from build123d import *

# Parameters (mm, degrees)
F1_DEPTH = 96.012
F3_D     = 15.875
F3_DEPTH = 31.75
F3_TIP   = 4.7693311635
F5_DEPTH = 56.897
F6_W     = 28.956
F6_H     = 13.716
F6_W_2   = 25.4
F6_H_2   = 19.304
F7_DEPTH = 50.801
F9_DEPTH = 56.897


with BuildPart() as f1:
    # F0 (on Right) → F1 (new body)
    with BuildSketch(Plane.YZ):
        Polygon((55.828121284, -27.6095795721), (55.828121284, 23.1904204279), (43.128121284, 23.1904204279), (-1.067878716, -21.0055795721), (-1.067878716, -27.6095795721), align=None)
    extrude(amount=F1_DEPTH)

    # F3
    with Locations(Plane.YZ.offset(96.012)):
        with Locations((36.524121284, -11.8615795721)):
            Hole(F3_D / 2, depth=F3_DEPTH)
            with Locations((0, 0, -(F3_DEPTH + F3_TIP / 2))):  # 118° drill point
                Cone(0, F3_D / 2, F3_TIP, mode=Mode.SUBTRACT)

    # F4 (on face) → F5 (cut, through all)
    with BuildSketch(Plane(origin=(0, 55.828121284, 0), x_dir=(-1, 0, 0), z_dir=(0, 1, 0))):
        Polygon((-96.012, 4.3944204279), (-77.216, 23.1904204279), (-96.012, 23.1904204279), align=None)
    extrude(amount=-F5_DEPTH, mode=Mode.SUBTRACT)

    # F6 (on face) → F7 (cut, through all)
    with BuildSketch(Plane(origin=(0, 0, -27.6095795721), x_dir=(1, 0, 0), z_dir=(0, 0, -1))):
        with Locations((39.878, -5.790121284)):
            Rectangle(F6_W, F6_H)
        with Locations((83.312, -8.584121284)):
            Rectangle(F6_W_2, F6_H_2)
    extrude(amount=-F7_DEPTH, mode=Mode.SUBTRACT)

    # F8 (on face) → F9 (cut, through all)
    with BuildSketch(Plane(origin=(0, 55.828121284, 0), x_dir=(-1, 0, 0), z_dir=(0, 1, 0))):
        Polygon((-16.2123730209, 4.3944204279), (0, 4.3944204279), (0, 23.1904204279), (-48.768, 23.1904204279), align=None)
    extrude(amount=-F9_DEPTH, mode=Mode.SUBTRACT)


solid = f1.part
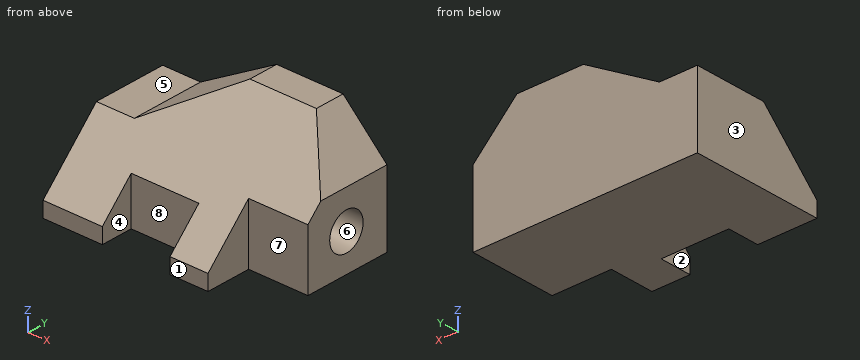
Build history of the part. All positions in model axes, mm. Face numbers are marked on the shaded views. A direction names the side the tool comes from. Give positions to 0.01 mm unless a question says otherwise; leave off trailing zeros. Order: outer loops, then holes, each group sorted by start corner. A loop starts at its lowest first (then second) coordinate and runs counter-clockwise, first axis right, second up. Notation, with made-up numbers: M 82.25,7.5 L 133.25,7.5 A21 cw 133.25,26.5 Z; hole C 43.5,15 d11. An arc over 180 degrees is marked long. Use one line per item in the form item = value.
Q1. Slice it at A-A, the plane y = 48. Write the cut outline in (x, z), and give its area (3 significant figures).
Conclusion:
outline = M 0,-27.61 L 96.01,-27.61 L 96.01,4.39 L 77.22,23.19 L 48.77,23.19 L 16.21,4.39 L 0,4.39 Z
area = 4,090 mm2
Q2. Pin check, flat tips, straight feed: P1, Ø10, axis at x = 61.5, z = 14.5, coming from the -Y side; P2, Ø18, axis at x = 11.5, y = 40, coming from the +Z side; P3, Ø6, axis at y = 35, z = 7.5, coming from the +X side. Stop position of each tip, or through.
Conclusion:
P1 = 29.44
P2 = 6.87
P3 = 95.91
Q3. Slice it at C-C, the plane x = 66. Write the cut outline in (y, z) (1 decimal).
Conclusion:
outline = M -1.1,-27.6 L 55.8,-27.6 L 55.8,23.2 L 43.1,23.2 L -1.1,-21 Z; hole C 36.5,-11.9 d15.9
Q4. Pull direction X, two halves, no side cores. Call the marked faces 1, 2, 3 and 4: released by +X, released by -X, zero draft, split by the parting line, or undercut.
Conclusion:
face_1 = zero draft
face_2 = undercut
face_3 = released by -X
face_4 = undercut
Q5. Wall check: probe 1 along Z at (x, y) = (86.5, 31); probe 2 along Y at (x, z) = (52, -15); probe 3 along X at (y, z) = (17.5, -13). Give the ranges that are in metal, low to high.
Conclusion:
probe_1 = -27.61 to -17.56, -6.16 to 11.06
probe_2 = 12.65 to 55.83
probe_3 = 0 to 70.61
Q6. Which spindle directions (+Z, -Z, +X, -X, +Y, -Y) get a long thin tool onto all of the face, cutting with end or side? Do the marked faces 5, 6, 7 and 8. Say none if no direction does.
Conclusion:
face_5 = +Z, -X, +Y, -Y
face_6 = +X
face_7 = +Z, -Z, +X, -Y
face_8 = +Z, -Z, -Y
Q7. Slice it at D-D, the plane z = 10. Write the cut outline in (x, y), and give its area (3 significant figures).
Conclusion:
outline = M 25.92,29.94 L 90.41,29.94 L 90.41,55.83 L 25.92,55.83 Z
area = 1,670 mm2
Q8. Slice it at B-B, the plane x = 8. Write the cut outline in (y, z).
Conclusion:
outline = M -1.07,-27.61 L 55.83,-27.61 L 55.83,4.39 L 24.33,4.39 L -1.07,-21.01 Z
